Verification items for the finished model (mm, model axes). A direction names the side the tool comes from. Coordinates: 2 decimals unless noted, no trailing zeros. Order: outer loops, then holes, each group sorted by start corner. A loop starts at its lowest first (then second) coordinate and runs counter-clockwise, first axis right, second up. Notation, with made-up numbers: (37.25, 67) - (88.25, 67) arc R36 cw to (88.25, 102) - close; hole circle Ø6 at (33.25, 24). An arc over 180 degrees is marked (long way). Answer as CSV lines item,"result". Start each with the question number.
1. Mould release check, pull along X, two halves, no side actions. Record for faces 3 (the cylindrical face through (0.54, -8.11, 2.44)), 4 (the cylindrical face through (-2.343, -4.93, 17.847)), 5 (the flat face through (8, -10, -8)): pulls with the +X half, pulls with the -X half, needs draft (parallel to the pull), parting line crosses it, or undercut.
2. Section check C-C (y = -14.25). Record the cut outline in (x, z).
3. Material ranges on L1, parallel to Z at x = 0, y = -9.5; L2, parallel to Z at x = 0, y = -12; L3, parallel to Y at x = 3.5, z = 11, recorded low to high. Write a range as [from, to].
4. Set-up check for faces 1 (the cylindrical face through (-2.17, -12.96, -9.76)), 2 (the flat face through (0, 0, -4)): record each of +Z, -Z, +X, -X, +Y, -Y from which the full face is reachable in a straight line by a thin tool's end or side.
5. Section check A-A (z = 0). Record the cut outline in (x, y).
6. Section check D-D (z = 6.5). Record the cut outline in (x, y).
7. Section check B-B (x = 0). Record the cut outline in (y, z), and give its area (3 significant figures).
8. Go/stop test with flat-tipped pins: pin 1 (2 mm diameter, centred on y = -3, z = 2.5, fed in from +X); pin 2 (6 mm diameter, centred on y = -9.5, z = 12, fed in from -X); pin 3 (8 mm diameter, centred on y = -10.5, z = -9, fed in from -X). Record where each tip stops, or that it passes through.
from build123d import *

# Parameters (mm, degrees)
F0_R     = 18
F0_R_2   = 10
F1_DEPTH = 10
F2_DEPTH = 16
F3_D     = 5


with BuildPart() as f1:
    # F0 (on Front) → F1 (new body)
    with BuildSketch(Plane.XZ):
        Circle(F0_R)
        Circle(F0_R_2, mode=Mode.SUBTRACT)
    extrude(amount=F1_DEPTH)

    # F0 (on Front) → F2 (join)
    with BuildSketch(Plane.XZ):
        Circle(F0_R_2)
    extrude(amount=F2_DEPTH)

    # F3 (through all)
    with Locations(Plane(origin=(0, 0, 0), x_dir=(1, 0, 0), z_dir=(0, 1, 0))):
        with Locations((0, 0)):
            Hole(F3_D / 2)


solid = f1.part
Evaluation:
1,face 3,"undercut"
1,face 4,"parting line crosses it"
1,face 5,"needs draft"
2,outline,"circle Ø20 at (0, 0); hole circle Ø5 at (0, 0)"
3,L1,"z = [-18, -2.5], [2.5, 18]"
3,L2,"z = [-10, -2.5], [2.5, 10]"
3,L3,"y = [-10, 0]"
4,face 1,"-Y"
4,face 2,"+Z, -Z, +X, -X, +Y"
5,outline,"(-18, -10) - (-10, -10) - (-10, -16) - (-2.5, -16) - (-2.5, 0) - (-18, 0) - close; (2.5, -16) - (10, -16) - (10, -10) - (18, -10) - (18, 0) - (2.5, 0) - close"
6,outline,"(-16.79, -10) - (-7.6, -10) - (-7.6, -16) - (7.6, -16) - (7.6, -10) - (16.79, -10) - (16.79, 0) - (-16.79, 0) - close"
7,outline,"(-16, -10) - (-10, -10) - (-10, -18) - (0, -18) - (0, -2.5) - (-16, -2.5) - close; (-16, 2.5) - (0, 2.5) - (0, 18) - (-10, 18) - (-10, 10) - (-16, 10) - close"
7,area,"400 mm²"
8,pin 1,"stops at x = 17.94"
8,pin 2,"stops at x = -15.59"
8,pin 3,"stops at x = -17.28"
